```python
from build123d import *

# Parameters (mm, degrees)
BOSS_EXTRUDE1_DEPTH = 20
CUT_EXTRUDE1_REACH  = 4
SKETCH2_R           = 3
SKETCH3_R           = 3
CUT_EXTRUDE2_DEPTH  = 20


with BuildPart() as part:
    # Sketch1 → Boss-Extrude1 (new body)
    with BuildSketch(Plane.XY):
        Polygon((0, 0), (15, 0), (15, 2), (2, 2), (2, 15), (0, 15), align=None)
    extrude(amount=BOSS_EXTRUDE1_DEPTH)

    # Sketch2 → Cut-Extrude1 (cut, up to next)
    with BuildSketch(Plane(origin=(0, 2, 0), x_dir=(1, 0, 0), z_dir=(0, 1, 0)), mode=Mode.PRIVATE) as cut_extrude1_sk1:
        with Locations((10, -10)):
            Circle(SKETCH2_R)
    cut_extrude1_tool1 = extrude(cut_extrude1_sk1.sketch, amount=-CUT_EXTRUDE1_REACH, mode=Mode.PRIVATE) & part.part
    add(cut_extrude1_tool1.solids().sort_by_distance((10, 2, 10))[0], mode=Mode.SUBTRACT)

    # Sketch3 → Cut-Extrude2 (cut)
    with BuildSketch(Plane(origin=(2, 0, 0), x_dir=(0, 0, -1), z_dir=(1, 0, 0))):
        with Locations((-10, 10)):
            Circle(SKETCH3_R)
    extrude(amount=-CUT_EXTRUDE2_DEPTH, mode=Mode.SUBTRACT)


solid = part.part
```
Model file for the job. Use its own axes, mm. A direction names the side the tool comes from. Coordinates: 2 decimals unless noted, no trailing zeros. Write each loop counter-clockwise with the first axis right and the second up, starting at its lowest first coordinate (ties: lowest second). Pieces come first, ordered by that corner, then holes. Notation, with made-up numbers: (88.25, 13.5) - (145.25, 13.5) arc R17 ccw to (145.25, 34.5) - close; hole circle Ø11 at (57.5, -18.5). An arc over 180 degrees is marked (long way). Use a Markdown table: item, result. Add a question column.
Item 1: Drill centre lines: line 1 along Y through (x, z) = (0.6, 10); line 2 along Z through (x, y) = (10, 1). Where is each one in solid material? Low to high.
Item 2: Band-saw the part on D-D, the plane x = 1.5. Write the cut outline in (y, z).
Item 3: Two-plate mould, pull along Z, no slides. Class faces 3 (the face through (1, 8.2, 12.4)), 4 (the face through (1, 5, 0)), 5 (the face through (1, 5, 20)), 6 (the face through (11.61, 1.01, 7.47)): pulls with the +Z half, pulls with the -Z half, needs draft (parallel to the pull), parting line crosses it, or undercut.
Item 4: Band-saw the part on C-C, the plane z = 12. Write the cut outline in (x, y), and give its area (3 significant figures).
Item 5: Band-saw the part on A-A, the plane x = 10. Write the cut outline in (y, z).
Item 6: 3-axis set-ups, long thin cutter, end or side, ignore diameter. For faces 1 (the face through (15, 1, 10)), 2 (the face through (2, 7, 8)): which of +Z, -Z, +X, -X, +Y, -Y reach the whole face in a straight line?
Item 7: Drop flat-ended pins along their axis: pin 1 (7 mm diameter, centred on y = 10, z = 10, fed in from +X); pin 2 (4 mm diameter, centred on x = 8, z = 7, fed in from +Y). Give the stop position or say it passes through.
A:
| question | item | result |
|---|---|---|
| 1 | line 1 | y = 0 to 7, 13 to 15 |
| 1 | line 2 | z = 0 to 7, 13 to 20 |
| 2 | outline | (0, 0) - (15, 0) - (15, 20) - (0, 20) - close; hole circle Ø6 at (10, 10) |
| 3 | face 3 | undercut |
| 3 | face 4 | pulls with the -Z half |
| 3 | face 5 | pulls with the +Z half |
| 3 | face 6 | undercut |
| 4 | outline | (0, 0) - (7.76, 0) - (7.76, 2) - (2, 2) - (2, 7.76) - (0, 7.76) - close; (0, 12.24) - (2, 12.24) - (2, 15) - (0, 15) - close; (12.24, 0) - (15, 0) - (15, 2) - (12.24, 2) - close |
| 4 | area | 38.1 mm² |
| 5 | outline | (0, 0) - (2, 0) - (2, 7) - (0, 7) - close; (0, 13) - (2, 13) - (2, 20) - (0, 20) - close |
| 6 | face 1 | +Z, -Z, +X, +Y, -Y |
| 6 | face 2 | +Z, -Z, +X, +Y |
| 7 | pin 1 | stops at x = 2 |
| 7 | pin 2 | stops at y = 2 |
